Check sheet for the drawn part. Datum: minimum x, y, z corner. Units: mm. Coordinates: 2 decimals unless noted, no trailing zeros. Loops run counter-clockwise (first coordinate to the right, second up) from the corner with the lowest first, then second, coordinate; pieces in that order, holes last. Notation, with made-up numbers: (26, 26) - (62, 26) arc R15 cw to (62, 50) - close; hole circle Ø4 at (1.5, -9.5). An arc over 180 degrees is marked (long way). Answer as CSV lines item,"result". Start each with the question number.
1. Gauge pin test, flat ends, axial feed: P1, Ø0.9, axis at x = 68.5, z = 1, coming from the +Y side; P2, Ø3, axis at x = 116.5, y = 11.5, coming from the -Z side. Record the tip position at first contact, or that the pin passes through.
2. Cross-section at B-B (y = 15). Enter the section's corners in (x, z).
3. Material ranges on line 1 (X direction, y = 25.5, z = 0.95) (1 decimal); line 2 (X direction, y = 26.5, z = 1.45) (1 decimal); line 3 (Y direction, x = 47.5, z = 1.45), recorded low to high. Write a range as [from, to].
4. Cross-section at C-C (z = 0.85). Enter the section's corners in (x, y), plus the area to 3 significant figures.
5. Cross-section at D-D (y = 5). Enter the section's corners in (x, z).
6. Cross-section at A-A (x = 47.5). Enter the section's corners in (y, z).
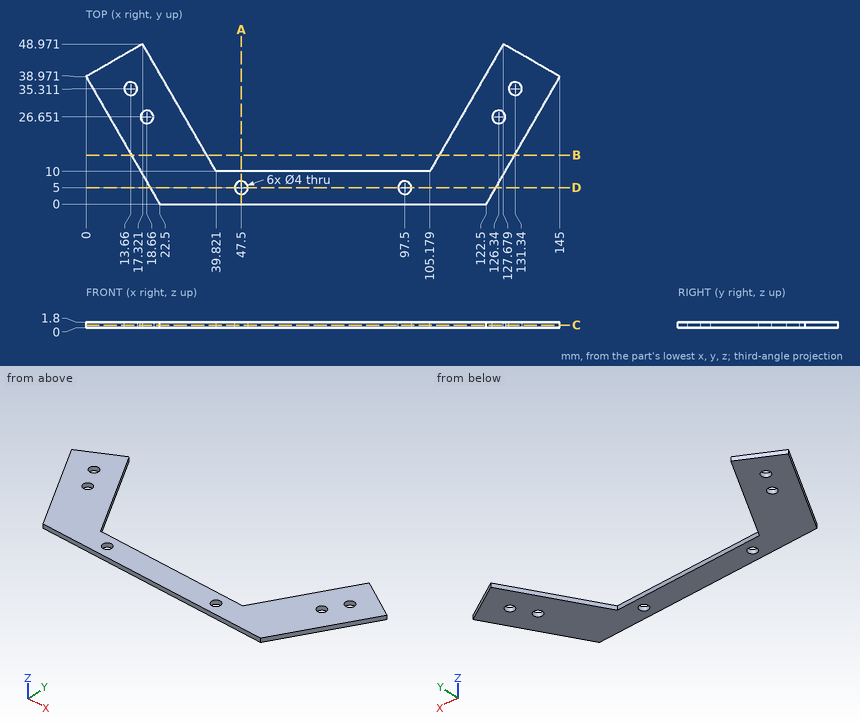
Values follow:
1,P1,"stops at y = 10"
1,P2,"stops at z = 0"
2,outline,"(13.84, 0) - (36.93, 0) - (36.93, 1.8) - (13.84, 1.8) - close; (108.07, 0) - (131.16, 0) - (131.16, 1.8) - (108.07, 1.8) - close"
3,line 1,"x = [7.8, 17], [20.3, 30.9], [114.1, 124.7], [128, 137.2]"
3,line 2,"x = [7.2, 16.7], [20.7, 30.3], [114.7, 124.3], [128.3, 137.8]"
3,line 3,"y = [0, 3], [7, 10]"
4,outline,"(0, 38.97) - (22.5, 0) - (122.5, 0) - (145, 38.97) - (127.68, 48.97) - (105.18, 10) - (39.82, 10) - (17.32, 48.97) - close; hole circle Ø4 at (13.66, 35.31); hole circle Ø4 at (18.66, 26.65); hole circle Ø4 at (47.5, 5); hole circle Ø4 at (97.5, 5); hole circle Ø4 at (126.34, 26.65); hole circle Ø4 at (131.34, 35.31)"
4,area,"2,550 mm²"
5,outline,"(19.61, 0) - (45.5, 0) - (45.5, 1.8) - (19.61, 1.8) - close; (49.5, 0) - (95.5, 0) - (95.5, 1.8) - (49.5, 1.8) - close; (99.5, 0) - (125.39, 0) - (125.39, 1.8) - (99.5, 1.8) - close"
6,outline,"(0, 0) - (3, 0) - (3, 1.8) - (0, 1.8) - close; (7, 0) - (10, 0) - (10, 1.8) - (7, 1.8) - close"
